Here's the drawing with two shaded views (mm, measured from the low corner). I have some questions. A direction names the side the tool comes from. Round coordinates to 2 decimals unless told otherwise and drop trailing zeros. Loops run counter-clockwise (first coordinate to the right, second up) from the corner with the lowest first, then second, coordinate; pieces in that order, holes last. Notation, with made-up numbers: (75, 30.5) -> (104, 30.5) arc R21 ccw to (104, 52.5) -> close; hole circle Ø9 at (35.5, 50). An arc over 180 degrees is marked (long way). Use a Markdown table: item, result.
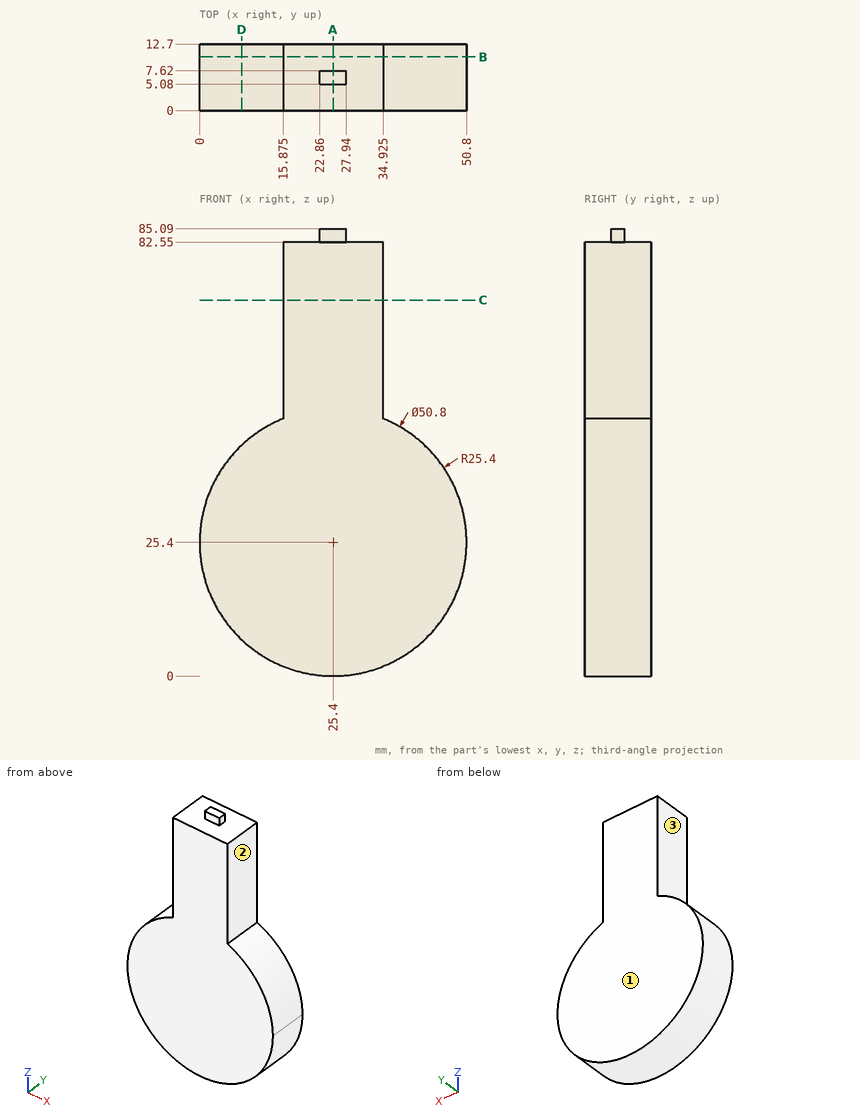
1. I want a section at D-D (x = 8). Please give me the cut outline in (y, z).
Answer sheet:
| item | result |
|---|---|
| outline | (0, 6.9) -> (12.7, 6.9) -> (12.7, 43.9) -> (0, 43.9) -> close |
2. Will these pins go through, and if not, where does the flat tip stop? pin 1 Ø6.5 at (y, z) = (5.5, 67.5) entering from +X (3 decimals); pin 2 Ø4 at (y, z) = (8.5, 73.5) entering from -X (3 decimals); pin 3 Ø0.8 at (y, z) = (6, 83) entering from +X.
Answer sheet:
| item | result |
|---|---|
| pin 1 | stops at x = 34.925 |
| pin 2 | stops at x = 15.875 |
| pin 3 | stops at x = 27.94 |
3. Which directions (+Z, -Z, +X, -X, +Y, -Y) give clear straight access to the entire face, cutting with the end or side of a thin tool? Please do the marked faces 1, 2 and 3.
Answer sheet:
| item | result |
|---|---|
| face 1 | +Z, -Z, +X, -X, +Y |
| face 2 | +Z, +X, +Y, -Y |
| face 3 | +Z, -X, +Y, -Y |
4. I want a section at C-C (z = 71.5). Please give me the cut outline in (x, y) (3 decimals).
Answer sheet:
| item | result |
|---|---|
| outline | (15.875, 0) -> (34.925, 0) -> (34.925, 12.7) -> (15.875, 12.7) -> close |
5. I want a section at B-B (y = 10.25). Please give me the cut outline in (x, z) (3 decimals).
Answer sheet:
| item | result |
|---|---|
| outline | (15.875, 48.946) arc R25.4 ccw (long way) to (50.8, 25.4) arc R25.4 ccw to (34.925, 48.946) -> (34.925, 82.55) -> (15.875, 82.55) -> close |
6. I need wall thicknesses on line 1 (X direction, y = 5, z = 81.5) (3 decimals); line 2 (Z direction, x = 25.5, y = 11.5); line 3 (Z direction, x = 25, y = 6). Which ranges of each line are inside material? Lowest first, please.
Answer sheet:
| item | result |
|---|---|
| line 1 | x = 15.875 to 34.925 |
| line 2 | z = 0 to 82.55 |
| line 3 | z = 0 to 85.09 |
7. I want a section at A-A (x = 25.4). Please give me the cut outline in (y, z), plus the area to 3 significant figures.
Answer sheet:
| item | result |
|---|---|
| outline | (0, 0) -> (12.7, 0) -> (12.7, 82.55) -> (7.62, 82.55) -> (7.62, 85.09) -> (5.08, 85.09) -> (5.08, 82.55) -> (0, 82.55) -> close |
| area | 1,050 mm² |
